CAD build for the part. Positions are in the model's coordinates, mm. Coordinates: 2 decimals unless noted, no trailing zeros. Write each loop counter-clockwise with the first axis right and the second up, starting at its lowest first coordinate (ties: lowest second). Pieces come first, ordered by that corner, then holes. Notation, with made-up numbers: (7.5, 77) - (36.5, 77) arc R28 cw to (36.5, 99) - close; hole circle Ø6 at (18, -23.75). An arc over 180 degrees is marked (long way). Answer in a Markdown table with one row per item. Add a question column.
Q1. Pin check, flat tips, straight feed: pin 1 (3 mm diameter, centred on x = -68.5, z = 7, fed in from -Y); pin 2 (1 mm diameter, centred on x = -150.5, z = 3, fed in from +Y); pin 3 (8.5 mm diameter, centred on y = 172.5, z = 16.5, fed in from -X). Stop position of each tip, or through.
Q2. Band-saw the part on B-B (y = 171). List the corners of the cut face in (x, z), and give its area (3 significant figures).
Q3. Band-saw the part on A-A (z = 3.75). List the corners of the cut face in (x, y), and give its area (3 significant figures).
Q4. Band-saw the part on D-D (y = 205). List the corners of the cut face in (x, z), and give its area (3 significant figures).
Q5. Band-saw the part on C-C (x = -217). List the corners of the cut face in (y, z).
Q6. Drill centre lines: line 1 along X through (y, z) = (168, 13.75); line 2 along X through (y, z) = (225, 16.25); line 3 along Y through (x, z) = (-196.5, 14). Where is each one in solid material? Low to high. Write a range as from..to.
```python
from build123d import *

# Parameters (mm, degrees)
F1_DEPTH = 19.05
F2_W     = 19.05
F2_H     = 7.62
F3_DEPTH = 254.001
F4_W     = 19.05
F4_H     = 7.62
F5_DEPTH = 254.001


with BuildPart() as f1:
    # F0 (on Top) → F1 (new body)
    with BuildSketch(Plane.XY):
        with BuildLine():
            ThreePointArc((0, 254), (-179.605122, 179.605122), (-254, 0))
            Line((-254, 0), (-220.285303, 0))
            Line((-220.285303, 0), (-234.95, 25.4))
            Line((-234.95, 25.4), (-184.15, 25.4))
            Line((-184.15, 25.4), (-198.814697, 0))
            Line((-198.814697, 0), (-165.1, 0))
            ThreePointArc((-165.1, 0), (-116.74333, 116.74333), (0, 165.1))
            Line((0, 165.1), (0, 198.814697))
            Line((0, 198.814697), (-25.4, 184.15))
            Line((-25.4, 184.15), (-25.4, 234.95))
            Line((-25.4, 234.95), (0, 220.285303))
            Line((0, 220.285303), (0, 254))
        make_face()
    extrude(amount=F1_DEPTH)

    # F2 (on Right) → F3 (cut, through all)
    with BuildSketch(Plane.YZ):
        with Locations((28.575, 15.24)):
            Rectangle(F2_W, F2_H)
    extrude(amount=-F3_DEPTH, mode=Mode.SUBTRACT)

    # F4 (on Front) → F5 (cut, through all)
    with BuildSketch(Plane.XZ):
        with Locations((-28.575, 15.24)):
            Rectangle(F4_W, F4_H)
    extrude(amount=-F5_DEPTH, mode=Mode.SUBTRACT)


solid = f1.part
```
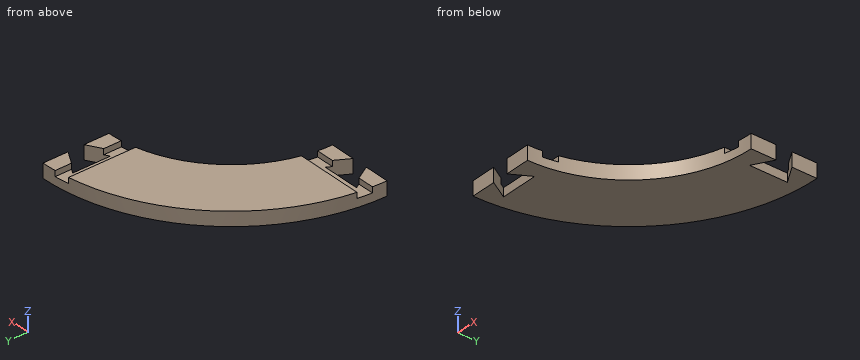
Checked values:
| question | item | result |
|---|---|---|
| 1 | pin 1 | stops at y = 149.53 |
| 1 | pin 2 | stops at y = 204.98 |
| 1 | pin 3 | stops at x = -190.28 |
| 2 | outline | (-187.82, 0) - (0, 0) - (0, 19.05) - (-19.05, 19.05) - (-19.05, 11.43) - (-38.1, 11.43) - (-38.1, 19.05) - (-187.82, 19.05) - close |
| 2 | area | 3,430 mm² |
| 3 | outline | (-254, 0) - (-220.29, 0) - (-234.95, 25.4) - (-184.15, 25.4) - (-198.81, 0) - (-165.1, 0) arc R165.1 cw to (0, 165.1) - (0, 198.81) - (-25.4, 184.15) - (-25.4, 234.95) - (0, 220.29) - (0, 254) arc R254 ccw to start |
| 3 | area | 27,400 mm² |
| 4 | outline | (-149.97, 0) - (-25.4, 0) - (-25.4, 11.43) - (-38.1, 11.43) - (-38.1, 19.05) - (-149.97, 19.05) - close |
| 4 | area | 2,280 mm² |
| 5 | outline | (25.4, 0) - (132.01, 0) - (132.01, 19.05) - (38.1, 19.05) - (38.1, 11.43) - (25.4, 11.43) - close |
| 6 | line 1 | x = -190.5..-38.1, -19.05..0 |
| 6 | line 2 | x = -117.86..-38.1, -8.17..0 |
| 6 | line 3 | y = 0..4.01, 38.1..160.95 |
